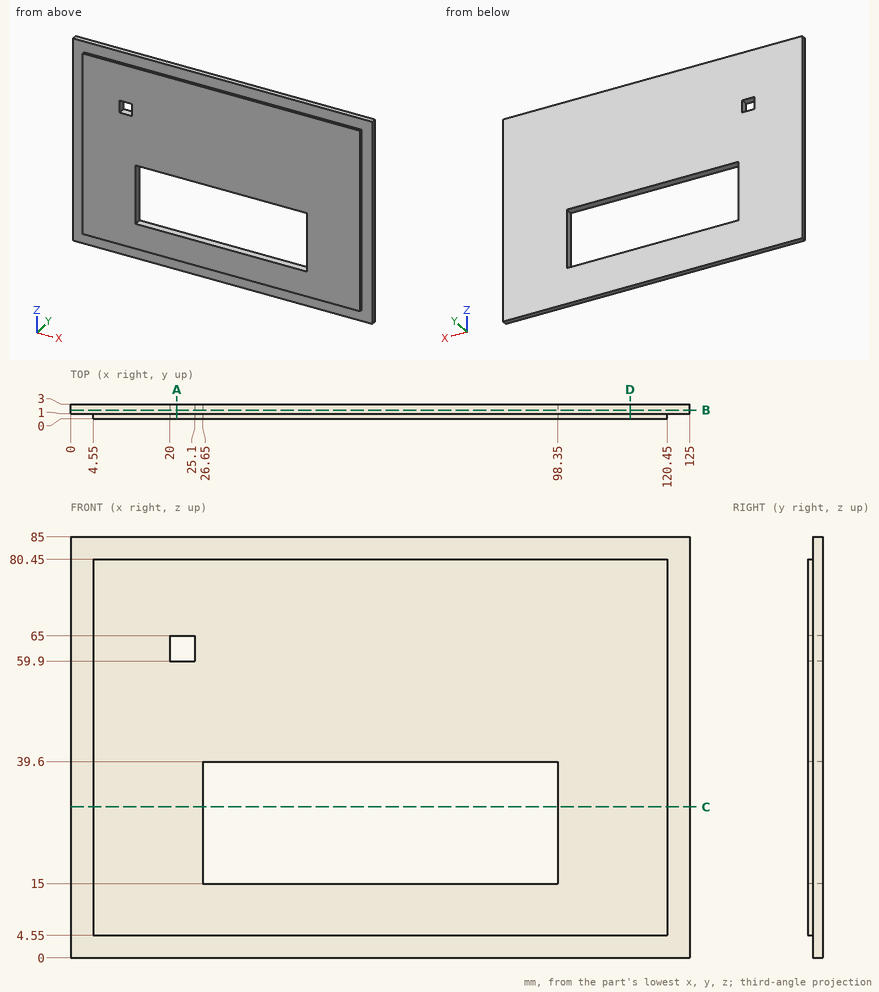
Source: three-view drawing plus pictorial views. Frame: mm from the lowest corner of the part. Round coordinates to 2 decimals unless told otherwise and drop trailing zeros. Loops run counter-clockwise (first coordinate to the right, second up) from the corner with the lowest first, then second, coordinate; pieces in that order, holes last.
Item 1: Section B-B, the plane y = 1.75. Output: boundary loops of the cut face in (x, z), plus the area to 3 significant figures.
Checked values:
outline: (0, 0) - (125, 0) - (125, 85) - (0, 85) - close; hole (20, 59.9) - (25.1, 59.9) - (25.1, 65) - (20, 65) - close; hole (26.65, 15) - (98.35, 15) - (98.35, 39.6) - (26.65, 39.6) - close
area: 8,840 mm2
Item 2: Section A-A, the plane x = 21.5. Output: boundary loops of the cut face in (y, z).
Checked values:
outline: (0, 4.55) - (1, 4.55) - (1, 0) - (3, 0) - (3, 59.9) - (0, 59.9) - close; (0, 65) - (3, 65) - (3, 85) - (1, 85) - (1, 80.45) - (0, 80.45) - close
Item 3: Contact query for flat-ended pins moving along their axis: P1, Ø0.5, axis at x = 69.5, y = 0.5, coming from the +Z side; P2, Ø0.5, axis at y = 0.5, z = 42, coming from the +X side; P3, Ø0.5, axis at x = 39.5, y = 0.5, coming from the -Z side. Output: stop coordinate, or through.
Checked values:
P1: stops at z = 80.45
P2: stops at x = 120.45
P3: stops at z = 4.55
Item 4: Line query: L1, parallel to X at y = 0.35, z = 21; L2, parallel to Z at x = 51.5, y = 0.6; L3, parallel to X at y = 1.6, z = 29. Output: solid intervals per line, ascending.
Checked values:
L1: x = 4.55 to 26.65, 98.35 to 120.45
L2: z = 4.55 to 15, 39.6 to 80.45
L3: x = 0 to 26.65, 98.35 to 125
Item 5: Section C-C, the plane z = 30.5. Output: boundary loops of the cut face in (x, y).
Checked values:
outline: (0, 1) - (4.55, 1) - (4.55, 0) - (26.65, 0) - (26.65, 3) - (0, 3) - close; (98.35, 0) - (120.45, 0) - (120.45, 1) - (125, 1) - (125, 3) - (98.35, 3) - close
Item 6: Section D-D, the plane x = 113. Output: boundary loops of the cut face in (y, z).
Checked values:
outline: (0, 4.55) - (1, 4.55) - (1, 0) - (3, 0) - (3, 85) - (1, 85) - (1, 80.45) - (0, 80.45) - close
